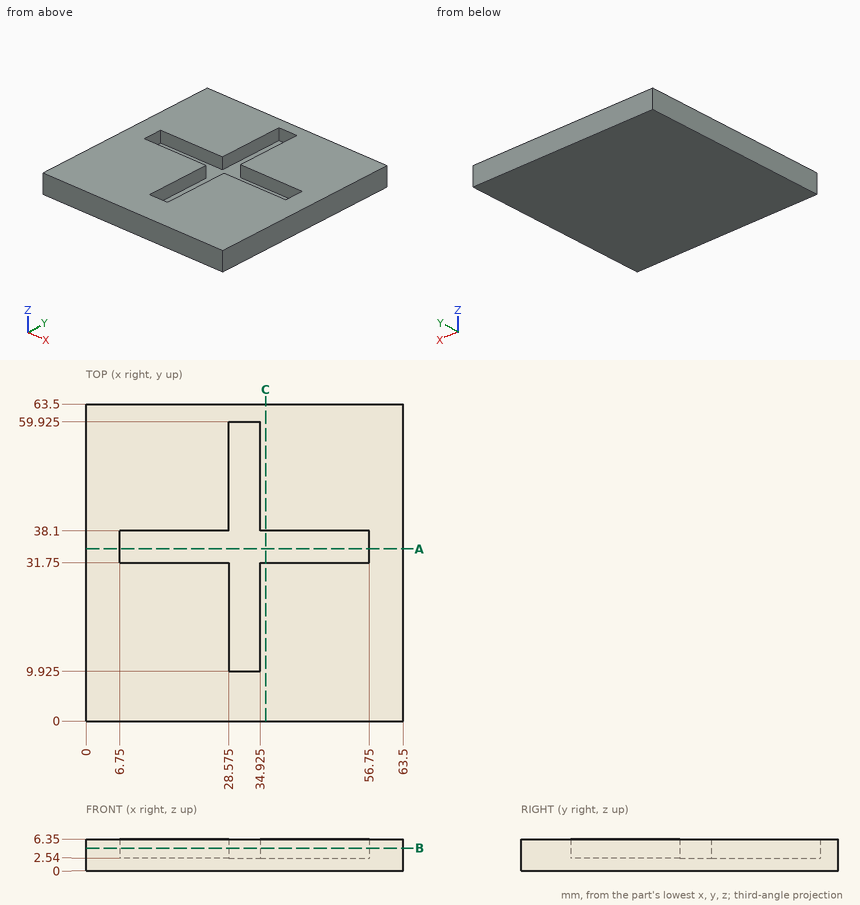
Source: three-view drawing plus pictorial views. Frame: mm from the lowest corner of the part. Give positions to 0.01 mm unless a question says otherwise; leave off trailing zeros. Loops run counter-clockwise (first coordinate to the right, second up) from the corner with the lowest first, then second, coordinate; pieces in that order, holes last. Notation, with made-up numbers: (-14, -29) -> (-5, -29) arc R11 cw to (-5, -23) -> close; hole circle Ø11 at (60, 12.25). An arc over 180 degrees is marked (long way). Put each result on its own line as item: value. Start each with the question number.
1) Cut plane B-B (z = 4.5). Return loops of the section in (x, y) (3 decimals), then the cut area to 3 significant figures.
2) Material intervals for probe 1 along Y at (x, z) = (18, 2.75); probe 2 along X at (y, z) = (17, 4.25) (3 decimals); probe 3 along Y at (x, z) = (29, 5) (3 decimals), sorted ascending.
3) Cut plane A-A (y = 34.5). Return loops of the section in (x, z), then the cut area to 3 significant figures.
4) Contact query for a flat-ended pin moving along its axis: P1, Ø3, axis at x = 32, z = 4.5, coming from the -Y side. Output: stop coordinate, or through.
5) Cut plane C-C (x = 36). Return loops of the section in (y, z), then the cut area to 3 significant figures.
Results are:
1. outline: (0, 0) -> (63.5, 0) -> (63.5, 63.5) -> (0, 63.5) -> close; hole (6.75, 31.75) -> (28.575, 31.75) -> (28.575, 9.925) -> (34.925, 9.925) -> (34.925, 31.75) -> (56.75, 31.75) -> (56.75, 38.1) -> (34.925, 38.1) -> (34.925, 59.925) -> (28.575, 59.925) -> (28.575, 38.1) -> (6.75, 38.1) -> close
1. area: 3,440 mm2
2. probe 1: y = 0 to 31.75, 38.1 to 63.5
2. probe 2: x = 0 to 28.575, 34.925 to 63.5
2. probe 3: y = 0 to 9.925, 59.925 to 63.5
3. outline: (0, 0) -> (63.5, 0) -> (63.5, 6.35) -> (56.75, 6.35) -> (56.75, 2.54) -> (6.75, 2.54) -> (6.75, 6.35) -> (0, 6.35) -> close
3. area: 213 mm2
4. P1: stops at y = 0
5. outline: (0, 0) -> (63.5, 0) -> (63.5, 6.35) -> (38.1, 6.35) -> (38.1, 2.54) -> (31.75, 2.54) -> (31.75, 6.35) -> (0, 6.35) -> close
5. area: 379 mm2
